Answer from the drawing. Dimensions are ordinates in mm from the lowest x, y and z of the part. A direction names the side the tool comes from. Round coordinates to 2 decimals unless told otherwise and drop trailing zeros. Loops run counter-clockwise (first coordinate to the right, second up) from the corner with the lowest first, then second, coordinate; pieces in that order, holes last.
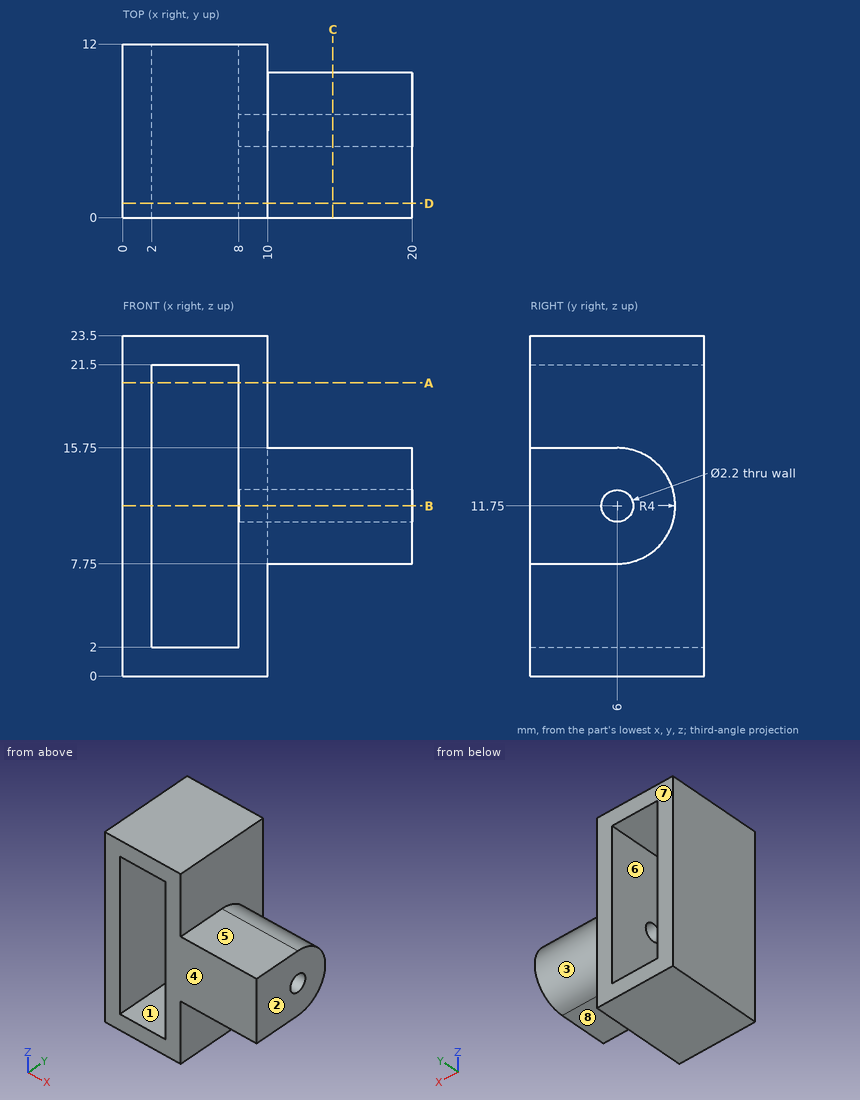
1. Which of the six approach directions +Z, -Z, +X, -X, +Y, -Y give full straight-line access (tool end or side, diameter ignored) to the marked faces 4, 5, 6, 7 and 8?
Answer key:
face 4: +Z, -Z, +X, -X, -Y
face 5: +Z, +X, +Y, -Y
face 6: +Y, -Y
face 7: +Z, -Z, +X, -X, +Y
face 8: -Z, +X, +Y, -Y
2. Find section C-C (x = 14.5). Write down the section's boundary in (y, z).
Answer key:
outline: (0, 7.75) - (6, 7.75) arc R4 ccw to (6, 15.75) - (0, 15.75) - close; hole circle Ø2.2 at (6, 11.75)
3. Find section A-A (z = 20.25). Write down the section's boundary in (x, y), then the cut area to 3 significant figures.
Answer key:
outline: (0, 0) - (2, 0) - (2, 12) - (0, 12) - close; (8, 0) - (10, 0) - (10, 12) - (8, 12) - close
area: 48.0 mm2
4. Determine the mould class of the marked faces 1, 2 and 3 for opening direction X: +X half, -X half, draft (parallel to the pull), parting line (faces both ways), or undercut.
Answer key:
face 1: undercut
face 2: +X half
face 3: draft
5. Find section B-B (z = 11.75). Write down the section's boundary in (x, y), then the cut area to 3 significant figures.
Answer key:
outline: (0, 0) - (2, 0) - (2, 12) - (0, 12) - close; (8, 0) - (20, 0) - (20, 4.9) - (8, 4.9) - close; (8, 7.1) - (20, 7.1) - (20, 10) - (10, 10) - (10, 12) - (8, 12) - close
area: 122 mm2
6. Consider probe 1 along X at (y, z) = (6.25, 2.5); probe 2 along Z at (x, y) = (10.5, 6); probe 3 along X at (y, z) = (2.75, 15.25). Determine where each line is inside the solid, lowest interval first.
Answer key:
probe 1: x = 0 to 2, 8 to 10
probe 2: z = 7.75 to 10.65, 12.85 to 15.75
probe 3: x = 0 to 2, 8 to 20
7. Given pin 1 (5 mm diameter, centred on x = 5, y = 4.5, fed in from -Z); pin 2 (6.5 mm diameter, centred on x = 14.5, y = 4, fed in from +Z); pin 3 (1.8 mm diameter, centred on x = 15, y = 2, fed in from -Z); pin 4 (5 mm diameter, centred on y = 10.5, z = 3.5, fed in from +X), each flat-ended and moving along its own axis, determine where each tip first touches the part or whether it passes through.
Answer key:
pin 1: stops at z = 0
pin 2: stops at z = 15.75
pin 3: stops at z = 7.75
pin 4: stops at x = 10
8. Find section D-D (y = 1). Write down the section's boundary in (x, z), then the cut area to 3 significant figures.
Answer key:
outline: (0, 0) - (10, 0) - (10, 7.75) - (20, 7.75) - (20, 15.75) - (10, 15.75) - (10, 23.5) - (0, 23.5) - close; hole (2, 2) - (8, 2) - (8, 21.5) - (2, 21.5) - close
area: 198 mm2
